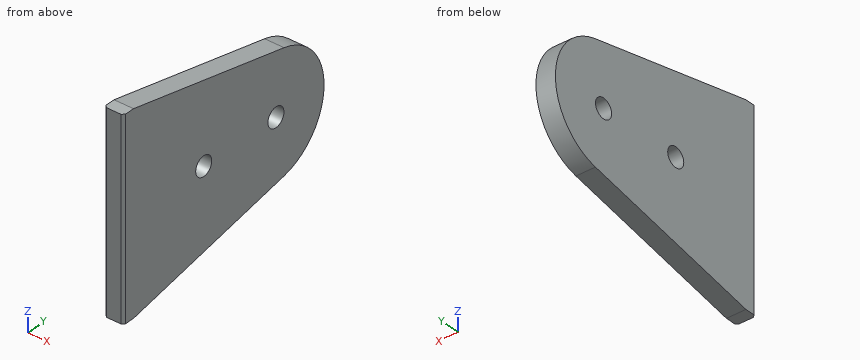
```python
from build123d import *

# Parameters (mm, degrees)
SKETCH1_R           = 4
BOSS_EXTRUDE1_DEPTH = 8
CHAMFER1_SIZE       = 1


with BuildPart() as part:
    # Sketch1 → Boss-Extrude1 (new body)
    with BuildSketch(Plane(origin=(0, 0, 0), x_dir=(0, 0, -1), z_dir=(1, 0, 0))):
        with BuildLine():
            Line((40, 0), (-40, 0))
            Line((-40, 0), (-40, 5))
            Line((-40, 5), (-24.482301542, 80.061315167))
            ThreePointArc((-24.482301542, 80.061315167), (0, 100), (24.482301542, 80.061315167))
            Line((24.482301542, 80.061315167), (40, 5))
            Line((40, 5), (40, 0))
        make_face()
        with Locations((0, 40)):
            Circle(SKETCH1_R, mode=Mode.SUBTRACT)
        with Locations((0, 76)):
            Circle(SKETCH1_R, mode=Mode.SUBTRACT)
    extrude(amount=BOSS_EXTRUDE1_DEPTH)

    # Chamfer1
    chamfer1_edges = [part.edges().sort_by_distance(p)[0] for p in [
        (8, 0, 0),
        (0, 0, 0),
    ]]
    chamfer(chamfer1_edges, length=CHAMFER1_SIZE)


solid = part.part
```
Source: CAD feature listing. Evaluate the final solid. Frame: model axes, mm. Coordinates: 2 decimals unless noted, no trailing zeros. Order: outer loops, then holes, each group sorted by start corner. A loop starts at its lowest first (then second) coordinate and runs counter-clockwise, first axis right, second up. Notation, with made-up numbers: (15.25, 0) - (56.25, 0) arc R25 cw to (56.25, 33) - close; hole circle Ø3 at (-29, 68.25). An arc over 180 degrees is marked (long way). One line per item, written item: value.
1) Contact query for flat-ended pins moving along their axis: pin 1 (4 mm diameter, centred on x = 2, y = 84.5, fed in from +Z); pin 2 (2 mm diameter, centred on x = 3.5, y = 24.5, fed in from -Z). Output: stop coordinate, or through.
Computed values:
pin 1: stops at z = 23.85
pin 2: stops at z = -36.18
2) Cut plane C-C on y = 76. Output: boundary loops of the cut face in (x, z), plus the area to 3 significant figures.
Computed values:
outline: (0, -25.32) - (8, -25.32) - (8, -4) - (0, -4) - close; (0, 4) - (8, 4) - (8, 25.32) - (0, 25.32) - close
area: 341 mm^2
3) Cut plane A-A on z = 0. Output: boundary loops of the cut face in (x, y).
Computed values:
outline: (0, 1) - (1, 0) - (7, 0) - (8, 1) - (8, 36) - (0, 36) - close; (0, 44) - (8, 44) - (8, 72) - (0, 72) - close; (0, 80) - (8, 80) - (8, 100) - (0, 100) - close
4) Cut plane D-D on z = 20. Output: boundary loops of the cut face in (x, y).
Computed values:
outline: (0, 1) - (1, 0) - (7, 0) - (8, 1) - (8, 90) - (0, 90) - close
5) Cut plane B-B on x = 4.5. Output: boundary loops of the cut face in (y, z).
Computed values:
outline: (0, -40) - (5, -40) - (80.06, -24.48) arc R25 ccw to (80.06, 24.48) - (5, 40) - (0, 40) - close; hole circle Ø8 at (40, 0); hole circle Ø8 at (76, 0)
6) Ray query, line 1 (Z direction, x = 2.5, y = 75); line 2 (Y direction, x = 2, z = 9.5); line 3 (Z direction, x = 4.75, y = 39.5). Return the intervals inside material, ascending. Write a range as [from, to].
Computed values:
line 1: z = [-25.53, -3.87], [3.87, 25.53]
line 2: y = [0, 98.12]
line 3: z = [-32.87, -3.97], [3.97, 32.87]
